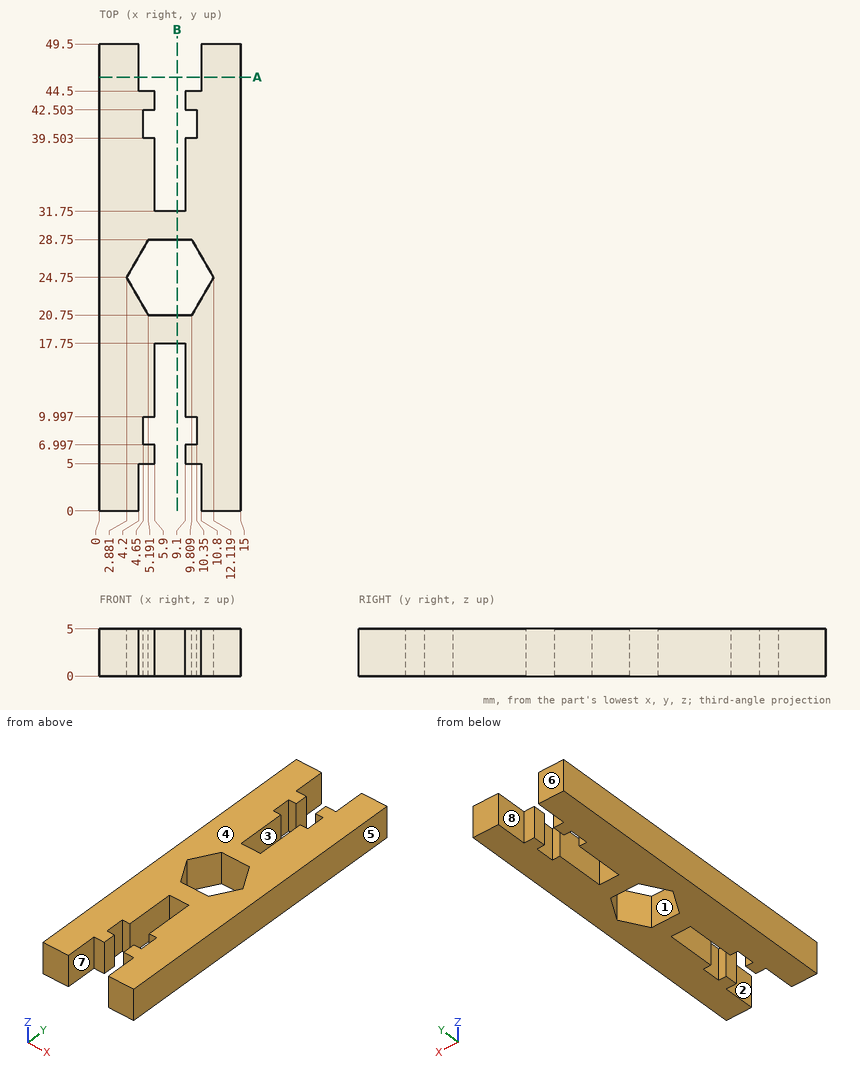
Geometry: see drawing. Coordinates: mm, zero at the bounding-box minimum. A direction names the side the tool comes from. Round coordinates to 2 decimals unless told otherwise and drop trailing zeros. Write each loop counter-clockwise with the first axis right and the second up, starting at its lowest first coordinate (ties: lowest second). Pieces come first, ordered by that corner, then holes.
1) Reachability of the marked faces 1, 2, 3 and 4 from +Z, -Z, +X, -X, +Y, -Y: full face, straight path, thin tool, end or side. Return the list, or none.
2) Cut plane B-B (x = 8.25). Return the cut outline in (y, z).
3) Contact query for flat-ended pins moving along their axis: P1, Ø0.6, axis at x = 5.5, z = 1.5, coming from the +Y side; P2, Ø0.8, axis at x = 4.5, z = 1.5, coming from the +Y side; P3, Ø1.6, axis at x = 7.5, z = 3, coming from the +Y side; P4, Ø3, axis at x = 9, z = 3.5, coming from the -Y side. Output: stop coordinate, or through.
4) Ray query, L1, parallel to X at y = 32.5, z = 2.4; L2, parallel to X at y = 4.5, z = 2.05; L3, parallel to Y at x = 5, z = 0.8 (1 decimal). Return the intervals inside material, ascending.
5) Draft query along X for the marked faces 5, 6, 7 and 8. Return one class per face: pulls with the +X half, pulls with the -X half, needs draft (parallel to the pull), parting line crosses it, or undercut.
6) Cut plane A-A (y = 46). Return the cut outline in (x, z), then the cut area to 3 significant figures.
Geometry says:
1. face 1: +Z, -Z
1. face 2: +Z, -Z, -Y
1. face 3: +Z, -Z, +Y
1. face 4: +Z, +X, -X, +Y, -Y
2. outline: (17.75, 0) - (20.75, 0) - (20.75, 5) - (17.75, 5) - close; (28.75, 0) - (31.75, 0) - (31.75, 5) - (28.75, 5) - close
3. P1: stops at y = 44.5
3. P2: stops at y = 49.5
3. P3: stops at y = 31.75
3. P4: stops at y = 5
4. L1: x = 0 to 5.9, 9.1 to 15
4. L2: x = 0 to 4.2, 10.8 to 15
4. L3: y = 5 to 7, 10 to 21.1, 28.4 to 39.5, 42.5 to 44.5
5. face 5: pulls with the +X half
5. face 6: needs draft
5. face 7: undercut
5. face 8: undercut
6. outline: (0, 0) - (4.2, 0) - (4.2, 5) - (0, 5) - close; (10.8, 0) - (15, 0) - (15, 5) - (10.8, 5) - close
6. area: 42.0 mm2
